Check sheet for the modelled part. Datum: model origin and axes. Units: mm. Face numbers are marked on the shaded views. A direction names the side the tool comes from. Give positions to 0.01 mm unless a question says otherwise; leave off trailing zeros. Write each loop counter-clockwise with the first axis right and the second up, starting at its lowest first coordinate (ties: lowest second). Pieces come first, ordered by that corner, then holes. Notation, with made-up numbers: M 36,87 L 65,87 A35 ccw 65,126 Z; hole C 60,-18 d6. An arc over 180 degrees is marked long. One line per item, written item: value. Start each with the question number.
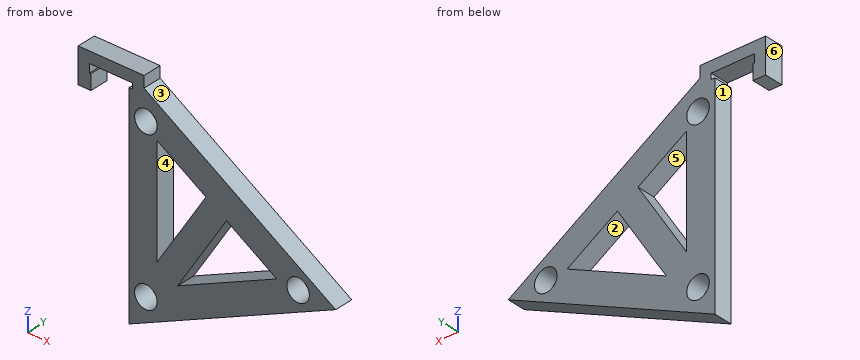
from build123d import *

# Parameters (mm, degrees)
F1_DEPTH = 10
F3_DEPTH = 25
F4_R     = 6
F5_DEPTH = 25
F6_W     = 2
F6_H     = 3
F7_DEPTH = 25


with BuildPart() as f1:
    # F0 (on Front) → F1 (new body)
    with BuildSketch(Plane.XZ):
        Polygon((-6, 0), (0, 0), (0, 8), (0, 12.5), (21, 12.5), (21, -102.735072), (131, -51.729484), (29, 12.5), (29, 18.5), (-6, 18.5), align=None)
        Polygon((0, 8), (0, 0), (0.75, 0), (0.75, 6.25), (0.75, 8), align=None)
    extrude(amount=F1_DEPTH)

    # F2 (on face) → F3 (cut)
    with BuildSketch(Plane.XZ.offset(10)):
        Polygon((61.977412, -25.99209), (36, -9.634093), (36, -67.245669), align=None)
        Polygon((99.665942, -49.724589), (72.907623, -32.874853), (46.886595, -74.197695), align=None)
    extrude(amount=-F3_DEPTH, mode=Mode.SUBTRACT)

    # F4 (on face) → F5 (cut)
    with BuildSketch(Plane.XZ.offset(10)):
        with Locations((30, -2.922298)):
            Circle(F4_R)
        with Locations((111, -50.5)):
            Circle(F4_R)
        with Locations((30, -86.28769)):
            Circle(F4_R)
    extrude(amount=-F5_DEPTH, mode=Mode.SUBTRACT)

    # F6 (on face) → F7 (cut)
    with BuildSketch(Plane.XZ.offset(10)):
        with Locations((22, 11)):
            Rectangle(F6_W, F6_H)
    extrude(amount=-F7_DEPTH, mode=Mode.SUBTRACT)


solid = f1.part
1) Material ranges on L1, parallel to Z at x = 34.5, y = -7.75; L2, parallel to Z at x = 2.5, y = -8.75; L3, parallel to Z at x = 30, y = -2, recorded low to high. Write a range as from..to.
2) Draft check along Z on the marked faces 1, 2, 3 and 4. Enter one of: released by +Z, released by -Z, zero draft, split by the parting line, or undercut.
3) Cross-section at D-D (y = -8.25). Record the boundary of the cut face in (x, z).
4) Cross-section at B-B (z = -20). Record the boundary of the cut face in (x, y).
5) Gauge pin test, flat ends, axial feed: pin 1 (3 mm diameter, centred on x = 114, z = -53, fed in from -Y); pin 2 (3 mm diameter, centred on x = 18.5, y = -7.5, fed in from -Z); pin 3 (3 mm diameter, centred on y = -2.5, z = -74, fed in from -X); pin 4 (1.3 mm diameter, centred on y = -6.5, z = 9.5, fed in from +X). Record the tip position at first contact, or that the pin passes through.
6) Cross-section at A-A (x = 86.5). Record the boundary of the cut face in (y, z), plus the area to 3 significant figures.
7) Tool access check on the marked faces 5 and 6. Record the directions out of +Z, -Z, +X, -X, +Y, -Y that give a thin tool (end or side, any length) a straight path to the whole face; none if there is none.
8) Cross-section at C-C (x = 26.5). Record the boundary of the cut face in (y, z), plus the area to 3 significant figures.
Data:
1. L1: z = -96.48..-90.26, -82.32..-6.89, 1.05..9.04
1. L2: z = 12.5..18.5
1. L3: z = -98.56..-92.29, -80.29..-8.92, 3.08..11.87
2. face 1: zero draft
2. face 2: undercut
2. face 3: released by +Z
2. face 4: undercut
3. outline: M -6,0 L 0.75,0 L 0.75,8 L 0,8 L 0,12.5 L 23,12.5 L 23,9.5 L 21,9.5 L 21,-102.74 L 131,-51.73 L 29,12.5 L 29,18.5 L -6,18.5 Z; hole C 30,-86.29 d12; hole C 30,-2.92 d12; hole M 36,-67.25 L 61.98,-25.99 L 36,-9.63 Z; hole M 46.89,-74.2 L 99.67,-49.72 L 72.91,-32.87 Z; hole C 111,-50.5 d12
4. outline: M 21,-10 L 36,-10 L 36,0 L 21,0 Z; M 52.46,-10 L 80.61,-10 L 80.61,0 L 52.46,0 Z
5. pin 1: passes through
5. pin 2: stops at z = 12.5
5. pin 3: stops at x = 21
5. pin 4: stops at x = 34.8
6. outline: M -10,-72.36 L 0,-72.36 L 0,-55.83 L -10,-55.83 Z; M -10,-41.43 L 0,-41.43 L 0,-23.71 L -10,-23.71 Z
6. area: 343 mm2
7. face 5: +Y, -Y
7. face 6: +Z, -Z, -X, +Y, -Y
8. outline: M -10,-100.18 L 0,-100.18 L 0,-91.16 L -10,-91.16 Z; M -10,-81.41 L 0,-81.41 L 0,-7.8 L -10,-7.8 Z; M -10,1.95 L 0,1.95 L 0,18.5 L -10,18.5 Z
8. area: 992 mm2
